from build123d import *

# Parameters (mm, degrees)
BOSS_EXTRUDE1_DEPTH     = 25.4
CUT_EXTRUDE1_DEPTH      = 110.310025801
CUT_EXTRUDE1_DEPTH_BACK = 110.310025801
SKETCH8_R               = 3.175
SKETCH9_R               = 3.175
CUT_EXTRUDE2_DEPTH      = 25.4
CUT_EXTRUDE3_DEPTH      = 75.639044044
CUT_EXTRUDE4_DEPTH      = 25.4
SKETCH14_W              = 33.446436581
SKETCH14_H              = 25.4
BOSS_EXTRUDE2_DEPTH     = 6.604
SKETCH15_W              = 83.98171134
SKETCH15_H              = 25.4
BOSS_EXTRUDE3_DEPTH     = 6.604
CUT_EXTRUDE5_DEPTH      = 79.566235631
FILLET11_R              = 12.7
CHAMFER1_SIZE           = 15.24
FILLET12_R              = 15.24
CUT_EXTRUDE6_DEPTH      = 1.27
CUT_EXTRUDE6_DEPTH_BACK = 1.27
CUT_EXTRUDE7_DEPTH      = 77.311629432
CUT_EXTRUDE7_DEPTH_BACK = 77.311629432
SKETCH21_W              = 1.27
SKETCH21_H              = 3.908978547


with BuildPart() as part:
    # Sketch2 → Boss-Extrude1 (new body)
    with BuildSketch(Plane(origin=(0, 0, 0), x_dir=(1, 0, 0), z_dir=(0, 1, 0))):
        Polygon((-0.93668344, 51.22431719), (-50.540816327, -34.692561236), (-46.141407275, -37.232561236), (-39.798130059, -26.24568281), (-35.398721007, -28.78568281), (-41.741998224, -39.772561236), (-37.342589173, -42.312561236), (-30.999311956, -31.32568281), (41.60831656, -31.32568281), (41.60831656, -5.92568281), (9.85831656, -5.92568281), (9.85831656, 38.52431719), (41.60831656, 38.52431719), (41.60831656, 51.22431719), align=None)
    extrude(amount=BOSS_EXTRUDE1_DEPTH)

    # Sketch8 → Cut-Extrude1 (cut, two sides: drawn at the far end of the back side and taken through both)
    with BuildSketch(Plane(origin=(0, 0, -51.22431719), x_dir=(-1, 0, 0), z_dir=(0, 0, -1)).offset(-CUT_EXTRUDE1_DEPTH_BACK)):
        with Locations((-25.7175, 12.7)):
            Circle(SKETCH8_R)
    extrude(amount=CUT_EXTRUDE1_DEPTH + CUT_EXTRUDE1_DEPTH_BACK, mode=Mode.SUBTRACT)

    # Sketch9 → Cut-Extrude2 (cut)
    with BuildSketch(Plane(origin=(-9.685065415, 0, -5.591675124), x_dir=(0.5000000000000036, 0, -0.8660254037844367), z_dir=(0.8660254037844366, 0, 0.5000000000000034))):
        with Locations((-48.965047516, 12.7)):
            Circle(SKETCH9_R)
    extrude(amount=-CUT_EXTRUDE2_DEPTH, mode=Mode.SUBTRACT)

    # Sketch11 → Cut-Extrude3 (cut, through all)
    with BuildSketch(Plane(origin=(-9.685065415, 0, -5.591675124), x_dir=(0.5000000000000036, 0, -0.8660254037844367), z_dir=(0.8660254037844366, 0, 0.5000000000000034))):
        with BuildLine():
            Line((-42.628493082, 25.4), (-52.778275903, 17.777577106))
            ThreePointArc((-52.778275903, 17.777577106), (-54.645562469, 15.538001034), (-55.315047516, 12.7))
            Line((-55.315047516, 12.7), (-55.315047516, 25.4))
            Line((-55.315047516, 25.4), (-42.628493082, 25.4))
        make_face()
    extrude(amount=-CUT_EXTRUDE3_DEPTH, mode=Mode.SUBTRACT)

    # Sketch12 → Cut-Extrude4 (cut)
    with BuildSketch(Plane(origin=(0, 25.4, 0), x_dir=(1, 0, 0), z_dir=(0, 1, 0))):
        Polygon((41.60831656, -18.62568281), (-23.666963538, -18.62568281), (-30.999311956, -31.32568281), (41.60831656, -31.32568281), align=None)
    extrude(amount=-CUT_EXTRUDE4_DEPTH, mode=Mode.SUBTRACT)

    # Sketch14 → Boss-Extrude2 (add)
    with BuildSketch(Plane(origin=(-9.685065415, 0, -5.591675124), x_dir=(0.5000000000000036, 0, -0.8660254037844367), z_dir=(0.8660254037844366, 0, 0.5000000000000034))):
        with Locations((-23.365274791, 12.7)):
            Rectangle(SKETCH14_W, SKETCH14_H)
    extrude(amount=BOSS_EXTRUDE2_DEPTH)

    # Sketch15 → Boss-Extrude3 (add)
    with BuildSketch(Plane(origin=(-22.883292569, 0, -13.211675124), x_dir=(-0.5000000000000002, 0, 0.8660254037844386), z_dir=(-0.8660254037844385, 0, -0.5000000000000001))):
        with Locations((-1.902362588, 12.7)):
            Rectangle(SKETCH15_W, SKETCH15_H)
    extrude(amount=BOSS_EXTRUDE3_DEPTH)

    # Sketch16 → Cut-Extrude5 (cut, through all)
    with BuildSketch(Plane(origin=(0, 25.4, 0), x_dir=(1, 0, 0), z_dir=(0, 1, 0))):
        Polygon((-0.93668344, 51.22431719), (-8.562325795, 51.22431719), (-6.655915206, 54.52631719), align=None)
    extrude(amount=-CUT_EXTRUDE5_DEPTH, mode=Mode.SUBTRACT)

    # Fillet11
    fillet11_edges = [part.edges().sort_by_distance(p)[0] for p in [
        (41.60831656, 25.4, -44.87431719),
        (41.60831656, 25.4, 12.27568281),
    ]]
    fillet(fillet11_edges, radius=FILLET11_R)

    # Chamfer1
    chamfer1_edges = [part.edges().sort_by_distance(p)[0] for p in [
        (9.85831656, 25.4, -16.29931719),
    ]]
    chamfer(chamfer1_edges, length=CHAMFER1_SIZE)

    # Fillet12
    fillet12_edges = [part.edges().sort_by_distance(p)[0] for p in [
        (-16.041321182, 12.7, 18.62568281),
        (-8.562325795, 12.7, -51.22431719),
    ]]
    fillet(fillet12_edges, radius=FILLET12_R)

    # Sketch19 → Cut-Extrude6 (cut, two sides: drawn at the far end of the back side and taken through both)
    with BuildSketch(Plane(origin=(0, 12.7, 0), x_dir=(1, 0, 0), z_dir=(0, 1, 0)).offset(-CUT_EXTRUDE6_DEPTH_BACK)):
        Polygon((-39.798130059, -26.24568281), (-35.398721007, -28.78568281), (-5.38168344, 23.20535135), (9.85831656, 23.20535135), (9.85831656, 25.74535135), (-5.38168344, 25.74535135), (-17.281047632, 25.74535135), (-17.281047632, 23.20535135), (-7.063084393, 23.20535135), align=None)
    extrude(amount=CUT_EXTRUDE6_DEPTH + CUT_EXTRUDE6_DEPTH_BACK, mode=Mode.SUBTRACT)

    # Sketch21 → Cut-Extrude7 (cut, two sides: drawn at the far end of the back side and taken through both)
    with BuildSketch(Plane(origin=(0, 25.4, 0), x_dir=(1, 0, 0), z_dir=(0, 1, 0)).offset(-CUT_EXTRUDE7_DEPTH_BACK)):
        with Locations((-16.708566929, 24.548624707)):
            Rectangle(SKETCH21_W, SKETCH21_H)
        with Locations((-11.628566929, 24.548624707)):
            Rectangle(SKETCH21_W, SKETCH21_H)
    extrude(amount=CUT_EXTRUDE7_DEPTH + CUT_EXTRUDE7_DEPTH_BACK, mode=Mode.SUBTRACT)


solid = part.part
Geometry check sheet. Reference: the model listing, model coordinates, mm. A direction names the side the tool comes from. Round coordinates to 2 decimals unless told otherwise and drop trailing zeros. Order: outer loops, then holes, each group sorted by start corner. A loop starts at its lowest first (then second) coordinate and runs counter-clockwise, first axis right, second up. Notation, with made-up numbers: M 51,20 L 66,20 A14 ccw 66,47 Z; hole C -12.75,46.25 d6. An arc over 180 degrees is marked long. Answer in a Markdown table with one row per item. Add a question column.
Item 1: Sectioned sample at D-D, the plane x = -9. Enter the section's corners in (y, z).
Item 2: Set-up check for faces 4 (the face through (23, 15, -38.524)), 5 (the face through (-26.91, 12.522, 30.754)), 6 (the face through (-9, 13, -23.205)), 7 (the face through (-22, 13.97, 1)): record each of +Z, -Z, +X, -X, +Y, -Y from which the full face is reachable in a straight line by a thin tool's end or side.
Item 3: Draft check along X on faces 1 (the face through (-13, 25.4, -5)), 2 (the face through (9.858, 5, -16)), 3 (the face through (-12.264, 13, -26)). Enter one of: released by +X, released by -X, zero draft, split by the parting line, or undercut.
Item 4: Sectioned sample at C-C, the plane y = 21. Enter the section's corners in (x, z), plus the area to 3 significant figures.
Item 5: Material ranges on L1, parallel to Y at x = -21.5, z = 3; L2, parallel to Z at x = 14.5, y = 19.75; L3, parallel to Z at x = 4.5, y = 12.75, recorded low to high. Write a range as [from, to].
Item 6: Sectioned sample at B-B, the plane z = -6.5. Enter the section's corners in (x, y), plus the area to 4 significant figures.
Item 7: Sectioned sample at A-A, the plane x = -27.5. Enter the section's corners in (y, z).
Item 8: Depth check by flat-ended pin: pin 1 Ø3 at (y, z) = (5, 21) entering from -X; pin 2 Ø1.3 at (x, y) = (-9.5, 13) entering from -Z; pin 3 Ø2 at (y, z) = (18, -24.5) entering from +X; pin 4 Ø10 at (x, z) = (13.5, -9) entering from -Y. Enter the tip coordinate at first touch or a pass-through.
Filled in:
| question | item | result |
|---|---|---|
| 1 | outline | M 0,-48.11 L 25.4,-48.11 L 25.4,18.73 L 0,18.73 Z; hole M 11.43,-25.75 L 13.97,-25.75 L 13.97,-23.21 L 11.43,-23.21 Z; hole M 11.43,-20.28 L 13.97,-20.28 L 13.97,-16.94 L 11.43,-16.94 Z |
| 2 | face 4 | +X, +Y |
| 2 | face 5 | +Z, +Y, -Y |
| 2 | face 6 | +X |
| 2 | face 7 | none |
| 3 | face 1 | zero draft |
| 3 | face 2 | released by +X |
| 3 | face 3 | undercut |
| 4 | outline | M -48.65,18.2 L -12.96,-43.6 A15.24 ccw 0.24,-51.22 L 38.52,-51.22 L 38.52,-38.52 L -0.98,-38.52 L -0.98,5.93 L 38.52,5.93 L 38.52,18.63 L -7.24,18.63 A15.24 cw -20.44,26.25 L -24.01,32.43 L -29.73,29.13 L -33.93,36.4 L -38.33,33.86 L -35.4,28.79 L -39.8,26.25 L -42.73,31.32 L -47.13,28.78 L -42.93,21.51 Z; hole M -17.34,-26.5 L -16.07,-26.5 L -16.07,-22.59 L -17.34,-22.59 Z; hole M -12.26,-26.5 L -10.99,-26.5 L -10.99,-22.59 L -12.26,-22.59 Z |
| 4 | area | 3,250 mm² |
| 5 | L1 | y = [0, 11.43], [13.97, 25.4] |
| 5 | L2 | z = [-51.22, -38.52], [5.93, 18.63] |
| 5 | L3 | z = [-51.22, -25.75], [-23.21, 18.63] |
| 6 | outline | M -34.38,0 L 9.86,0 L 9.86,10.16 L -5.38,25.4 L -34.38,25.4 Z; hole M -18.12,11.43 L -15.03,11.43 L -15.03,13.97 L -18.12,13.97 Z |
| 6 | area | 1,000 mm² |
| 7 | outline | M 0,-18.42 L 25.4,-18.42 L 25.4,30.41 L 0,30.41 Z; hole M 11.43,7.67 L 13.97,7.67 L 13.97,15.1 L 11.43,15.1 Z |
| 8 | pin 1 | stops at x = -46.4 |
| 8 | pin 2 | stops at z = -48.22 |
| 8 | pin 3 | stops at x = 3.02 |
| 8 | pin 4 | stops at y = 0 |
